Drawing for the job (mm, zero at the part's lowest x, y, z). A direction names the side the tool comes from. Give positions to 0.01 mm unless a question says otherwise; leave off trailing zeros. Order: outer loops, then holes, each group sorted by start corner. A loop starts at its lowest first (then second) coordinate and runs counter-clockwise, first axis right, second up. Notation, with made-up numbers: (74, -23) - (126, -23) arc R29 cw to (126, 6) - close; hole circle Ø4 at (10.5, 27.25). An arc over 180 degrees is marked (long way). Use CSV: the item, a comma, the result in double quotes. Start each with the question number.
(1) Drop flat-ended pins along their axis: pin 1 Ø1.9 at (x, y) = (83.5, 9) entering from +Z (3 decimals); pin 2 Ø5.5 at (x, z) = (57, 24.5) entering from +Y; pin 3 Ø2 at (y, z) = (29.5, 21.5) entering from -X. Give the stop position or say it passes through.
(2) Band-saw the part on A-A, the plane x = 27. Give the cut face in (y, z).
(3) Tool access for the marked faces 5, 6, 7 and 8: list every direction of +Z, -Z, +X, -X, +Y, -Y with a clear straight run to the whole face (end or side of a thin tool).
(4) Probe L1, parallel to Z at x = 63, y = 14.5; L2, parallel to Z at x = 106, y = 14.5 (1 decimal); L3, parallel to Z at x = 107.5, y = 13 (1 decimal). List the from-to ranges inside material, lowest first.
(5) Pull direction X, two halves, no side cores. Call the marked faces 1, 2, 3 and 4: +X half, -X half, draft (parallel to the pull), parting line (faces both ways), or undercut.
(6) Band-saw the part on C-C, the plane y = 24. Give the cut face in (x, z), then the cut area to 3 significant figures.
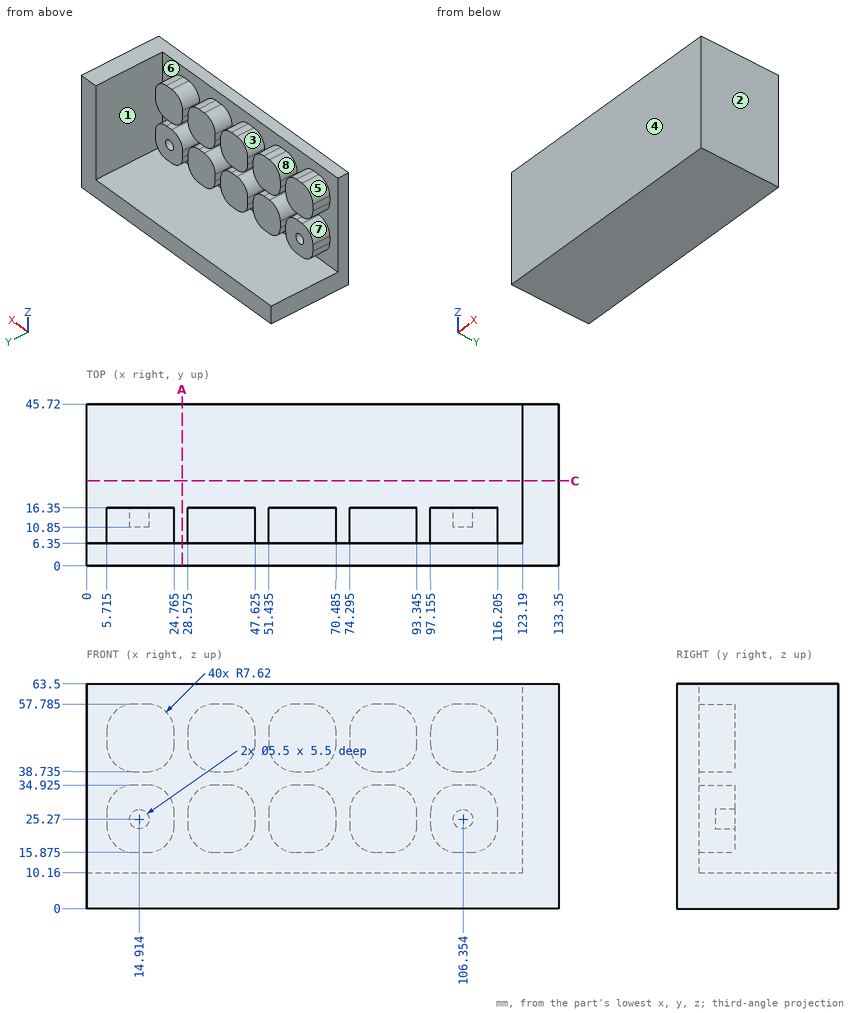
Answer block:
1,pin 1,"stops at z = 57.785"
1,pin 2,"stops at y = 16.35"
1,pin 3,"stops at x = 123.19"
2,outline,"(0, 0) - (45.72, 0) - (45.72, 10.16) - (6.35, 10.16) - (6.35, 63.5) - (0, 63.5) - close"
3,face 5,"+Z, -X, +Y"
3,face 6,"+Y"
3,face 7,"-X, +Y"
3,face 8,"+Z, +Y"
4,L1,"z = 0 to 10.16, 15.88 to 34.92, 38.74 to 57.78"
4,L2,"z = 0 to 10.2, 15.9 to 22.5, 28 to 34.9, 38.7 to 57.8"
4,L3,"z = 0 to 10.2, 15.9 to 22.8, 27.8 to 34.9, 38.7 to 57.8"
5,face 1,"undercut"
5,face 2,"+X half"
5,face 3,"undercut"
5,face 4,"draft"
6,outline,"(0, 0) - (133.35, 0) - (133.35, 63.5) - (123.19, 63.5) - (123.19, 10.16) - (0, 10.16) - close"
6,area,"1,900 mm2"
